```python
from build123d import *

# Parameters (mm, degrees)
SKETCH2_R           = 6.35
BOSS_EXTRUDE1_DEPTH = 1.5875
SKETCH3_W           = 6.35
SKETCH3_H           = 6.35
SKETCH3_W_2         = 3.175
SKETCH3_H_2         = 3.175
BOSS_EXTRUDE2_DEPTH = 3.175


with BuildPart() as part:
    # Sketch2 → Boss-Extrude1 (new body)
    with BuildSketch(Plane.XY):
        Circle(SKETCH2_R)
    extrude(amount=BOSS_EXTRUDE1_DEPTH)

    # Sketch3 → Boss-Extrude2 (add)
    with BuildSketch(Plane(origin=(0, 0, 0), x_dir=(-1, 0, 0), z_dir=(0, 0, -1))):
        Rectangle(SKETCH3_W, SKETCH3_H)
        Rectangle(SKETCH3_W_2, SKETCH3_H_2, mode=Mode.SUBTRACT)
    extrude(amount=BOSS_EXTRUDE2_DEPTH)


solid = part.part
```
The listing builds one solid part. Answer for the finished solid, in the listing's coordinates (mm). A direction names the side the tool comes from. Round coordinates to 2 decimals unless told otherwise and drop trailing zeros. Write each loop counter-clockwise with the first axis right and the second up, starting at its lowest first coordinate (ties: lowest second). Pieces come first, ordered by that corner, then holes. Notation, with made-up numbers: (-20.75, 82) -> (37.25, 82) arc R17 ccw to (37.25, 106) -> close; hole circle Ø2 at (-3.75, -39.5). An arc over 180 degrees is marked (long way). Write item = value, one per line.
1) Section D-D on z = 0.9 is taken. Write down the section's boundary in (x, y).
Check values:
outline = circle Ø12.7 at (0, 0)
2) Straight lines are drawn through the part: line 1 along X through (y, z) = (1.25, -2.6) (1 decimal); line 2 along Z through (x, y) = (-5, 0.5); line 3 along Y through (x, z) = (-1.75, -0.25) (3 decimals). For each, find the intervals that lie inside material, in ascending order. Write a range as [from, to].
Check values:
line_1 = [-3.2, -1.6], [1.6, 3.2]
line_2 = [0, 1.59]
line_3 = [-3.175, 3.175]
3) Section B-B on z = -0.75 is taken. Write down the section's boundary in (x, y) (1 decimal), plus the area to 3 significant figures.
Check values:
outline = (-3.2, -3.2) -> (3.2, -3.2) -> (3.2, 3.2) -> (-3.2, 3.2) -> close; hole (-1.6, -1.6) -> (1.6, -1.6) -> (1.6, 1.6) -> (-1.6, 1.6) -> close
area = 30.2 mm²
4) Which of the six approach directions +Z, -Z, +X, -X, +Y, -Y give full straight-line access (tool end or side, diameter ignored) to faces 4 (the flat face through (-3.175, 0, -2)), 5 (the flat face through (0, 1.588, -2)), 6 (the flat face through (0, -3.175, -2))?
Check values:
face_4 = -Z, -X, +Y, -Y
face_5 = -Z
face_6 = -Z, +X, -X, -Y
5) Given pin 1 (1.6 mm diameter, centred on y = -0.5, z = -1.5, fed in from -X) (3 decimals); pin 2 (2.5 mm diameter, centred on y = 0, z = -1.5, fed in from +X) (3 decimals); pin 3 (1 mm diameter, centred on x = 0.5, z = -2, fed in from -Y) (3 decimals), each flat-ended and moving along its own axis, determine where each tip first touches the part or whether it passes through.
Check values:
pin_1 = -3.175
pin_2 = 3.175
pin_3 = -3.175
6) For a pull along Y with two mould halves and no side action, classify faces 1 (the flat face through (0, 3.175, -2)), 2 (the flat face through (3.175, 0, -2)), 3 (the flat face through (-1.588, 0, -2)) as released by +Y, released by -Y, zero draft, split by the parting line, or undercut.
Check values:
face_1 = released by +Y
face_2 = zero draft
face_3 = undercut
